For this review, take the finished solid that the model builds, in its own axes (mm). Face numbers are marked on the shaded views. A direction names the side the tool comes from. Give positions to 0.01 mm unless a question says otherwise; leave off trailing zeros. Order: outer loops, then holes, each group sorted by start corner. A loop starts at its lowest first (then second) coordinate and runs counter-clockwise, first axis right, second up. Notation, with made-up numbers: (65, 37) -> (93, 37) arc R20 cw to (93, 69) -> close; hole circle Ø8 at (77, 60). An arc over 180 degrees is marked (long way). Return JSON: item names as keys, results as strings. Group by question number.
1) Add section C-C (z = 16). Give the boundary of the cut face in (x, y).
2) Add section A-A (y = 0). Give the boundary of the cut face in (x, z).
3) The part is to be moulded in two halves that separate along Y. For the marked faces 3, 4 and 5, say which applies: released by +Y, released by -Y, zero draft, split by the parting line, or undercut.
4) For the marked faces 1 and 2, list the 3-axis set-ups (+Z, -Z, +X, -X, +Y, -Y) from which the entire face can be reached by the end or side of a thin tool; tool diameter is ignored.
5) Add section D-D (z = 11). Give the boundary of the cut face in (x, y), then the cut area to 3 significant figures.
6) Insertion check: P1, Ø1, axis at x = -3, y = -8.5, coming from the +Z side; P2, Ø12, axis at x = 14.5, z = 25, coming from the +Y side; P3, Ø5, axis at x = -13.5, z = 12, coming from the -Y side; P4, Ø6, axis at x = -9, y = -5, coming from the -Z side. Each pin has a flat end and moves straight along its axis. Give the tip position at first contact, or say it passes through.
7) To check wall thickness, follow line 1 along Y through (x, z) = (0, 26); line 2 along Y through (x, z) = (0, 15.9); line 3 along X through (y, z) = (-14.5, 23). State the ranges of each line that lie inside material, in increasing order.
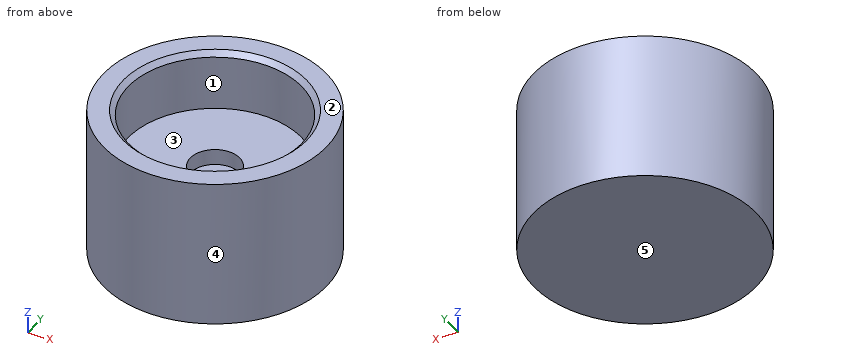
Autodesk Inventor part; units mm, degrees
ref_plane "YZ Plane" through (0, 0, 0) normal (1, 0, 0) x (0, 1, 0)
ref_plane "XZ Plane" through (0, 0, 0) normal (0, 1, 0) x (-1, 0, 0)
ref_plane "XY Plane" through (0, 0, 0) normal (0, 0, 1) x (1, 0, 0)
sketch "Sketch1" plane through (0, 0, 0) normal (0, 0, 1) x (1, 0, 0)
  circle A0 centre (0, 0) radius 22.5
  dimension "d0" = 45
extrude "Extrusion1" add sketch "Sketch1" along normal blind 30
sketch "Sketch2" plane through (0, 0, 30) normal (0, 0, 1) x (1, 0, 0)
  circle A0 centre (0, 0) radius 17.5
  dimension "d3" = 35
extrude "Extrusion2" cut sketch "Sketch2" against normal blind 12
chamfer "Chamfer1" distance 1 angle 45 1 edges at (-17.5, 0, 30)
sketch "Sketch3" plane through (0, 0, 18) normal (0, 0, 1) x (1, 0, 0)
  circle A0 centre (0, 0) radius 5
  circle A1 centre (0, 0) radius 5
  point P0 (0, 0)
extrude "Extrusion3" cut sketch "Sketch3" against normal blind 3.2
Evaluation:
{
 "1": {"outline": "circle Ø45 at (0, 0); hole circle Ø10 at (0, 0)"},
 "2": {"outline": "(-22.5, 0) -> (22.5, 0) -> (22.5, 30) -> (18.5, 30) -> (17.5, 29) -> (17.5, 18) -> (5, 18) -> (5, 14.8) -> (-5, 14.8) -> (-5, 18) -> (-17.5, 18) -> (-17.5, 29) -> (-18.5, 30) -> (-22.5, 30) -> close"},
 "3": {"face 3": "undercut", "face 4": "split by the parting line", "face 5": "zero draft"},
 "4": {"face 1": "+Z", "face 2": "+Z, +X, -X, +Y, -Y"},
 "5": {"outline": "circle Ø45 at (0, 0)", "area": "1,590 mm^2"},
 "6": {"P1": "z = 18", "P2": "y = 20.83", "P3": "y = -19.63", "P4": "z = 0"},
 "7": {"line 1": "-22.5 to -17.5, 17.5 to 22.5", "line 2": "-22.5 to -5, 5 to 22.5", "line 3": "-17.2 to -9.8, 9.8 to 17.2"}
}
